CAD build for the part. Positions are in the model's coordinates, mm. A direction names the side the tool comes from. Coordinates: 2 decimals unless noted, no trailing zeros. Order: outer loops, then holes, each group sorted by start corner. A loop starts at its lowest first (then second) coordinate and runs counter-clockwise, first axis right, second up. Notation, with made-up numbers: (48.25, 39.5) - (53.25, 39.5) arc R21 ccw to (53.25, 49.5) - close; hole circle Ø9 at (20, 18.25). An arc over 180 degrees is marked (long way). Use one line per item in the form item = value.
Autodesk Inventor part; units mm, degrees
ref_plane "YZ Plane" through (0, 0, 0) normal (1, 0, 0) x (0, 1, 0)
ref_plane "XZ Plane" through (0, 0, 0) normal (0, 1, 0) x (-1, 0, 0)
ref_plane "XY Plane" through (0, 0, 0) normal (0, 0, 1) x (1, 0, 0)
sketch "Szkic1" plane through (0, 0, 0) normal (0, 1, 0) x (-1, 0, 0)
  line L0 (0, 0) -> (0, -43.18)
  line L1 (0, -43.18) -> (15.875, -38.9263)
  line L2 (0, -43.18) -> (16.435, -43.18) construction
  line L3 (0, 0) -> (15.875, -4.2537)
  line L4 (0, 0) -> (18.9194, 0) construction
  line L5 (15.875, -21.59) -> (15.875, -4.2537)
  line L6 (15.875, -21.59) -> (15.875, -38.9263)
  dimension "d0" = 43.18
  dimension "d2" = 15
  dimension "d3" = 15
  dimension "d4" = 15.875
extrude "Wyciągnięcie proste1" add sketch "Szkic1" along normal blind 177.8
sketch "Szkic2" plane through (0, 0, 0) normal (1, 0, 0) x (0, 0, -1)
  line L0 (0, 0) -> (43.18, 0)
  line L1 (0, 177.8) -> (43.18, 177.8)
  line L2 (43.18, 0) -> (43.18, 177.8)
  line L3 (0, 0) -> (0, 177.8)
  point P0 (12.065, 9.525)
  point P1 (12.065, 55.245)
  point P2 (12.065, 122.555)
  point P3 (12.065, 168.275)
  point P4 (31.115, 168.275)
  point P5 (31.115, 122.555)
  point P6 (31.115, 55.245)
  point P7 (31.115, 9.525)
  dimension "d7" = 45.72
  dimension "d8" = 67.31
  dimension "d9" = 45.72
  dimension "d10" = 9.525
  dimension "d12" = 19.05
  dimension "d13" = 19.05
  dimension "d14" = 19.05
  dimension "d15" = 19.05
  dimension "d18" = 12.065
  dimension "d19" = 12.065
  dimension "d20" = 12.065
  dimension "d21" = 12.065
  dimension "d48" = 9.525
  dimension "d49" = 45.72
  dimension "d50" = 67.31
  dimension "d51" = 45.72
hole "Otwór1" at (0, 9.525, -12.065) at (0, 55.245, -12.065) at (0, 122.555, -12.065) at (0, 168.275, -12.065) at (0, 168.275, -31.115) at (0, 122.555, -31.115) at (0, 55.245, -31.115) at (0, 9.525, -31.115) direction (-1, 0, 0) diameter 6.756 depth 30 tip angle 118 counterbore diameter 11.113 counterbore depth 8.89
sketch "Szkic3" plane through (-15.875, 0, -38.9263) normal (-1, 0, 0) x (0, 0, 1)
  line L0 (34.6726, 0) -> (34.6726, 177.8)
  line L1 (0, 0) -> (0, 177.8)
  line L2 (0, 177.8) -> (34.6726, 177.8)
  point P0 (38.9263, 0)
  point P1 (17.3366, 106.4)
  point P2 (17.3366, 71.4)
  dimension "d29" = 17.336
  dimension "d31" = 17.336
  dimension "d34" = 35
  dimension "d35" = 71.4
hole "Otwór2" at (-15.875, 106.4, -21.5897) at (-15.875, 71.4, -21.5897) direction (1, 0, 0) diameter 6.401 depth 22.931 tip angle 118
sketch "Szkic4" plane through (-15.875, 0, -38.9263) normal (-1, 0, 0) x (0, 0, 1)
  line L0 (0, 0) -> (0, 177.8)
  line L1 (34.6726, 0) -> (34.6726, 177.8)
  circle A0 centre (26.8613, 122.555) radius 5.5565
  circle A1 centre (7.8113, 122.555) radius 3.378
  circle A2 centre (26.8613, 55.245) radius 3.378
  circle A3 centre (7.8113, 55.245) radius 3.378
  arc A4 (13.9583, 122.555) -> (20.7143, 122.555) centre (17.3363, 122.555) ccw
  arc A5 (20.7143, 158.344) -> (13.9583, 158.344) centre (17.3363, 158.344) ccw
  arc A6 (20.7143, 55.245) -> (13.9583, 55.245) centre (17.3363, 55.245) ccw
  arc A7 (13.9583, 19.456) -> (20.7143, 19.456) centre (17.3363, 19.456) ccw
  line L2 (20.7143, 158.344) -> (20.7143, 122.555)
  line L3 (13.9583, 122.555) -> (13.9583, 158.344)
  line L4 (21.3048, 122.555) -> (20.7143, 122.555)
  line L5 (11.1893, 122.555) -> (7.8113, 122.555)
  line L6 (20.7143, 55.245) -> (20.7143, 19.456)
  line L7 (13.9583, 19.456) -> (13.9583, 55.245)
  point P0 (38.9263, 0)
  dimension "d45" = 34.6726
  dimension "d54" = 6.756
  dimension "d55" = 6.756
  dimension "d56" = 6.756
  dimension "d57" = 6.756
  dimension "d66" = 35.789
  dimension "d67" = 35.789
  dimension "d68" = 0
  dimension "d69" = 35.789
  dimension "d70" = 35.789
extrude "Wyciągnięcie proste2" cut sketch "Szkic4" against normal blind 177.8 contours A4 L3 A5 L2 | L6 A7 L7 A6
sketch "Szkic7" plane through (0, 0, 0) normal (1, 0, 0) x (0, 0, -1)
  arc A0 (18.212, 19.456) -> (24.968, 19.456) centre (21.59, 19.456) ccw
  arc A1 (16.0335, 19.456) -> (27.1465, 19.456) centre (21.59, 19.456) ccw
  arc A2 (24.968, 55.245) -> (18.212, 55.245) centre (21.59, 55.245) ccw
  arc A3 (27.1465, 55.245) -> (16.0335, 55.245) centre (21.59, 55.245) ccw
  line L0 (16.0335, 19.456) -> (16.0335, 55.245)
  line L1 (27.1465, 19.456) -> (27.1465, 55.245)
  arc A4 (24.968, 158.344) -> (18.212, 158.344) centre (21.59, 158.344) ccw
  arc A5 (16.0335, 122.555) -> (27.1465, 122.555) centre (21.59, 122.555) ccw
  arc A6 (27.1465, 158.344) -> (16.0335, 158.344) centre (21.59, 158.344) ccw
  line L2 (16.0335, 122.555) -> (16.0335, 158.344)
  line L3 (27.1465, 122.555) -> (27.1465, 158.344)
  point P0 (0, 0)
  dimension "d71" = 11.113
  dimension "d72" = 11.113
  dimension "d73" = 11.113
  dimension "d74" = 11.113
extrude "Wyciągnięcie proste4" cut sketch "Szkic7" against normal blind 8.89
fillet "Zaokrąglenie1" radius 4 8 edges at (-4.445, 51.3558, -16.0335) (-4.445, 58.1074, -16.8275) (-4.445, 58.1074, -26.3525) (-4.445, 51.3558, -27.1465) (-4.445, 119.6926, -16.8275) (-4.445, 119.6926, -26.3525) (-4.445, 126.4442, -16.0335) (-4.445, 126.4442, -27.1465)
sketch "Szkic8" plane through (-15.875, 0, -38.9263) normal (-1, 0, 0) x (0, 0, 1)
  arc A0 (13.9583, 19.456) -> (20.7143, 19.456) centre (17.3363, 19.456) ccw
  line L0 (17.3363, 19.456) -> (17.3363, 202.652)
  line L1 (17.3363, 19.456) -> (17.3363, -13.8574)
  line L2 (0, 177.8) -> (34.6726, 177.8)
  line L3 (0, 0) -> (34.6726, 0)
  point P0 (38.9263, 0)
  point P1 (17.3363, 6.5)
  point P2 (17.3363, 171.3)
  dimension "d78" = 6.5
  dimension "d79" = 6.5
hole "Otwór3" at (-15.875, 6.5, -21.59) at (-15.875, 171.3, -21.59) direction (1, 0, 0) diameter 4.978 depth 19.05 tip angle 118
equation "\"d67\" = d66"
equation "\"d69\" = d66"
equation "\"d70\" = d69"
properties part number "dovetail" material "Aluminium 6061"
Item 1: Two-plate mould, pull along Y, no slides. Class faces 1 (the face through (-8, 177.8, -21)), 2 (the face through (-7.83, 87.66, -2.1)), 3 (the face through (-12, 141, -18.212)): +Y half, -Y half, draft (parallel to the pull), parting line (faces both ways), or undercut.
Derived:
face_1 = +Y half
face_2 = draft
face_3 = undercut
Item 2: Cut at A-A, the plane y = 71.4. Write the cut outline in (x, z) (3 decimals), plus the area to 3 significant figures.
Derived:
outline = (-15.875, -38.926) - (0, -43.18) - (0, -24.79) - (-15.875, -24.79) - close; (-15.875, -18.389) - (0, -18.389) - (0, 0) - (-15.875, -4.254) - close
area = 516 mm²
Item 3: Drill centre lines: line 1 (Z direction, x = -3.5, y = 171.3); line 2 (Y direction, x = -12, z = -11.5); line 3 (Y direction, x = -1, z = -15). Where is each one in solid material? Low to high. Write a range as [from, to].
Derived:
line_1 = [-42.24, -35.78], [-26.45, -24.08], [-19.1, -16.73], [-7.4, -0.94]
line_2 = [0, 6.19], [12.86, 51.91], [58.58, 119.22], [125.89, 164.94], [171.61, 177.8]
line_3 = [0, 4.81], [14.24, 48.37], [59.97, 117.83], [129.43, 163.56], [172.99, 177.8]
Item 4: Cut at B-B, the plane y = 153.5. Write the cut outline in (x, z) (1 decimal).
Derived:
outline = (-15.9, -38.9) - (0, -43.2) - (0, -27.1) - (-8.9, -27.1) - (-8.9, -25) - (-15.9, -25) - close; (-15.9, -18.2) - (-8.9, -18.2) - (-8.9, -16) - (0, -16) - (0, 0) - (-15.9, -4.3) - close
Item 5: Drop flat-ended pins along their axis: pin 1 (7.5 mm diameter, centred on x = -13, y = 144.5, fed in from -Z); pin 2 (5 mm diameter, centred on x = -12, y = 73.5, fed in from +Z); pin 3 (6 mm diameter, centred on x = -5, y = 61, fed in from +Z). Give the stop position or say it passes through.
Derived:
pin_1 = -40.7
pin_2 = -2.55
pin_3 = -0.54
Item 6: 3-axis set-ups, long thin cutter, end or side, ignore diameter. For faces 4 (the face through (-4.507, 56.824, -36.442)), 5 (the face through (-7.83, 87.66, -41.08)), 6 (the face through (-12, 38, -18.212)): which of +Z, -Z, +X, -X, +Y, -Y reach the whole face in a straight line?
Derived:
face_4 = +X
face_5 = -Z, -X, +Y, -Y
face_6 = +X, -X
Item 7: Cut at C-C, the plane z = -21.59. State how many separate pieces and enclosed holes the cut face has, plus the area to 3 significant figures.
Derived:
separate_pieces = 7
enclosed_holes = 0
area = 1,030 mm²
